from build123d import *

# Parameters (mm, degrees)
F0_W          = 127
F0_H          = 12.7
F0_R          = 3.175
F1_DEPTH      = 9.525
F2_R          = 5.08
F5_W          = 101.6
F5_H          = 19.05
F6_DEPTH      = 3.175
F6_DEPTH_BACK = 3.175
F7_SIZE       = 3.17499
F8_R          = 9.52499


# Not quite as in the source:
# - a fillet or chamfer is up to 0.001 mm smaller than in the source, because OpenCascade refuses the exact size


with BuildPart() as f1:
    # F0 (on Front) → F1 (new body)
    with BuildSketch(Plane.XZ):
        Rectangle(F0_W, F0_H)
        with Locations((-57.15, 0)):
            Circle(F0_R, mode=Mode.SUBTRACT)
        with Locations((57.15, 0)):
            Circle(F0_R, mode=Mode.SUBTRACT)
    extrude(amount=F1_DEPTH)

    # F2
    f2_edges = [f1.edges().sort_by_distance(p)[0] for p in [
        (-63.5, -4.7625, 6.35),
        (-63.5, -4.7625, -6.35),
        (63.5, -4.7625, 6.35),
        (63.5, -4.7625, -6.35),
    ]]
    fillet(f2_edges, radius=F2_R)

    # F5 (on face) → F6 (join, two sides)
    with BuildSketch(Plane(origin=(0, -4.7625, 0), x_dir=(-1, 0, 0), z_dir=(0, 1, 0))) as f6_sk:
        with Locations((-12.7, 0)):
            Rectangle(F5_W, F5_H)
        with BuildLine():
            ThreePointArc((-57.1005828679, 4.1822632775), (-52.9233760572, 0.0930895553), (-57.0553988218, -4.0417364798))
            ThreePointArc((-57.0553988218, -4.0417364798), (-61.2736674525, 0.0472116417), (-57.1005828679, 4.1822632775))
        make_face(mode=Mode.SUBTRACT)
    extrude(amount=F6_DEPTH)
    extrude(f6_sk.sketch, amount=-F6_DEPTH_BACK)

    # F7 (size 3.175 in the source; OpenCascade refuses exactly that, so slightly less here)
    f7_edges = [f1.edges().sort_by_distance(p)[0] for p in [
        (-38.1, -4.7625, 9.525),
        (-38.1, -4.7625, -9.525),
    ]]
    chamfer(f7_edges, length=F7_SIZE)

    # F8 (radius 9.525 in the source; OpenCascade refuses exactly that, so slightly less here)
    f8_edges = [f1.edges().sort_by_distance(p)[0] for p in [
        (63.5, -4.7625, 9.525),
        (63.5, -4.7625, -9.525),
    ]]
    fillet(f8_edges, radius=F8_R)


solid = f1.part
Input: part model. Units: mm. Frame: model coordinates. A direction names the side the tool comes from. Round coordinates to 2 decimals unless told otherwise and drop trailing zeros. Loops run counter-clockwise (first coordinate to the right, second up) from the corner with the lowest first, then second, coordinate; pieces in that order, holes last. Notation, with made-up numbers: (-13.5, -4.75) -> (1.5, -4.75) arc R8 cw to (1.5, 7.25) -> close; hole circle Ø6 at (26.5, 3.25). An arc over 180 degrees is marked (long way). Answer as a JSON object with one key per item and string values. Group by question number.
1) Pin query (flat end, axial travel): pin 1 (5 mm diameter, centred on x = 57.15, z = 0, fed in from +Y); pin 2 (4 mm diameter, centred on y = -7, z = -4.5, fed in from -X); pin 3 (1.5 mm diameter, centred on x = 20.5, z = -8, fed in from -Y). Return the tip coordinate at first contact, or that it passes through.
2) Reachability of faces 1 (the cylindrical face through (60.62, -0.8, -5.85)), 2 (the flat face through (-13.8, -0.5, 6.35)), 3 (the flat face through (-1, 0, 0)), 4 (the cylindrical face through (60.62, -0.8, 5.85)) from +Z, -Z, +X, -X, +Y, -Y: full face, straight path, thin tool, end or side. Return the list, or none.
3) Ray query, L1, parallel to Z at x = -57.15, y = -4 (3 decimals); L2, parallel to X at y = -0.75, z = -1.5; L3, parallel to X at y = -6.5, z = 0.5. Return the intervals inside material, ascending.
4) Draft query along Z for faces 5 (the cylindrical face through (60.62, -8.74, 5.85)), 6 (the cylindrical face through (-62.051, -4.829, -4.822)), 7 (the cylindrical face through (53.98, -4.7, 0.14)), 8 (the cylindrical face through (-54.12, -4.7, 0.95)). Return one class per face: +Z half, -Z half, draft (parallel to the pull), parting line (faces both ways), or undercut.
5) Section query B-B on x = -57.15. Output: boundary loops of the cut face in (y, z) (3 decimals).
6) Section query A-A on y = -5.25. State how many separate pieces and enclosed holes the cut face has, plus the area to 3 significant figures.
Reply:
{
 "1": {"pin 1": "passes through", "pin 2": "stops at x = -63.35", "pin 3": "stops at y = -7.94"},
 "2": {"face 1": "-Z, +X, +Y", "face 2": "+Z, -X", "face 3": "+Z, -Z, +X, -X, +Y", "face 4": "+Z, +X, +Y"},
 "3": {"L1": "z = -6.35 to -3.175, 3.175 to 6.35", "L2": "x = -63.49 to -59.95, -54.35 to 54.35, 59.95 to 63.38", "L3": "x = -63.5 to -60.29, -54.01 to 54.01, 60.29 to 63.49"},
 "4": {"face 5": "+Z half", "face 6": "-Z half", "face 7": "undercut", "face 8": "undercut"},
 "5": {"outline": "(-9.525, -6.35) -> (0, -6.35) -> (0, -3.175) -> (-9.525, -3.175) -> close; (-9.525, 3.175) -> (0, 3.175) -> (0, 6.35) -> (-9.525, 6.35) -> close"},
 "6": {"separate pieces": "1", "enclosed holes": "2", "area": "2,130 mm2"}
}
